Check sheet for the modelled part. Datum: model origin and axes. Units: mm. Give positions to 0.01 mm unless a question says otherwise; leave off trailing zeros. Loops run counter-clockwise (first coordinate to the right, second up) from the corner with the lowest first, then second, coordinate; pieces in that order, holes last. Notation, with made-up numbers: (-33.5, -16) -> (4.5, -16) arc R13 ccw to (4.5, -10) -> close; hole circle Ø7 at (26.25, 81). An arc over 180 degrees is marked (long way). Write each question's results on one line, items separated by ' | '. Start each with the question number.
Item 1: Gauge pin test, flat ends, axial feed: pin 1 Ø1.4 at (x, y) = (2.5, 82.5) entering from -Z; pin 2 Ø2.5 at (x, z) = (2, 138.5) entering from -Y; pin 3 Ø1.4 at (x, y) = (3.5, 82.5) entering from +Z. Record the tip position at first contact, or that the pin passes through.
Item 2: Cross-section at A-A on z = 131.5. Enter the section's corners in (x, y).
Item 3: Scan lines: line 1 along Z through (x, y) = (1.05, 108.5); line 2 along Z through (x, y) = (0.8, 84.5); line 3 along Y through (x, z) = (2, 19). Record each from-to range of solid material in increasing order.
Item 4: Cross-section at B-B on y = 91.5. Enter the section's corners in (x, z).
Item 5: Cross-section at C-C on x = 1.75. State how many separate pieces and enclosed holes the cut face has, then the cut area to 3 significant figures.
from build123d import *

# Parameters (mm, degrees)
SKETCH1_R           = 4
SKETCH1_R_2         = 1.5
SKETCH1_W           = 13.2
SKETCH1_H           = 5.2
BOSS_EXTRUDE1_DEPTH = 5


with BuildPart() as part:
    # Sketch1 → Boss-Extrude1 (new body)
    with BuildSketch(Plane(origin=(0, 0, 0), x_dir=(0, 0, -1), z_dir=(1, 0, 0))):
        Polygon((-135.781354304, 106.733539226), (-135.781354304, 139.733539226), (-8.651354304, 139.733539226), (-8.651354304, 106.733539226), (-3.651354304, 106.733539226), (-3.651354304, 93.533539226), (-8.651354304, 93.533539226), (-8.651354304, 85.833539226), (-19.651354304, 85.833539226), (-19.651354304, 87.133539226), (-22.151354304, 87.133539226), (-22.151354304, 85.833539226), (-29.008589557, 85.833539226), (-29.008589557, 82.833539226), (-22.151354304, 82.833539226), (-22.151354304, 81.533539226), (-19.651354304, 81.533539226), (-19.651354304, 82.833539226), (-8.651354304, 82.833539226), (-8.651354304, 75.133539226), (-3.651354304, 75.133539226), (-3.651354304, 61.933539226), (-8.651354304, 61.933539226), (-8.651354304, 53.933539226), (-135.781354304, 53.933539226), (-135.781354304, 61.933539226), (-140.781354304, 61.933539226), (-140.781354304, 75.133539226), (-135.781354304, 75.133539226), (-135.781354304, 82.833539226), (-124.781354304, 82.833539226), (-124.781354304, 81.533539226), (-122.281354304, 81.533539226), (-122.281354304, 82.833539226), (-115.424119051, 82.833539226), (-115.424119051, 85.833539226), (-122.281354304, 85.833539226), (-122.281354304, 87.133539226), (-124.781354304, 87.133539226), (-124.781354304, 85.833539226), (-135.781354304, 85.833539226), (-135.781354304, 93.533539226), (-140.781354304, 93.533539226), (-140.781354304, 106.733539226), align=None)
        with Locations((-72.216354304, 84.333539226)):
            Circle(SKETCH1_R, mode=Mode.SUBTRACT)
        with Locations((-81.216354304, 84.333539226)):
            Circle(SKETCH1_R_2, mode=Mode.SUBTRACT)
        with Locations((-63.216354304, 84.333539226)):
            Circle(SKETCH1_R_2, mode=Mode.SUBTRACT)
        with Locations((-72.216354304, 106.733539226)):
            Circle(SKETCH1_R_2, mode=Mode.SUBTRACT)
        with Locations((-56.416354304, 106.733539226)):
            Rectangle(SKETCH1_W, SKETCH1_H, mode=Mode.SUBTRACT)
        with Locations((-88.016354304, 106.733539226)):
            Rectangle(SKETCH1_W, SKETCH1_H, mode=Mode.SUBTRACT)
    extrude(amount=BOSS_EXTRUDE1_DEPTH)


solid = part.part
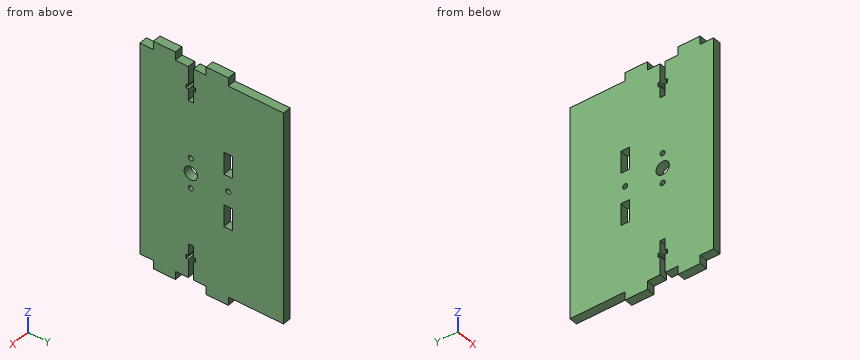
Answer sheet:
1) pin 1: stops at z = 8.65 | pin 2: stops at y = 61.93 | pin 3: stops at z = 135.78
2) outline: (0, 53.93) -> (5, 53.93) -> (5, 82.83) -> (0, 82.83) -> close; (0, 85.83) -> (5, 85.83) -> (5, 139.73) -> (0, 139.73) -> close
3) line 1: z = 8.65 to 49.82, 63.02 to 81.42, 94.62 to 135.78 | line 2: z = 29.01 to 61.73, 64.71 to 68.22, 76.21 to 79.73, 82.71 to 115.42 | line 3: y = 53.93 to 82.83, 85.83 to 139.73
4) outline: (0, 8.65) -> (5, 8.65) -> (5, 135.78) -> (0, 135.78) -> close
5) separate pieces: 1 | enclosed holes: 6 | area: 10,800 mm²
